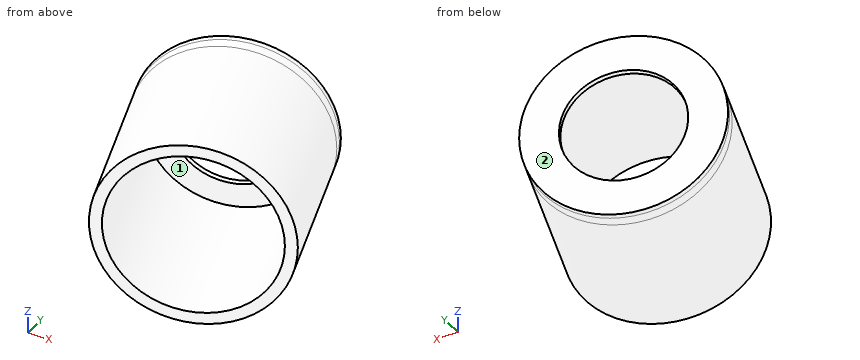
Autodesk Inventor part; units mm, degrees
ref_plane "YZ Plane" through (0, 0, 0) normal (1, 0, 0) x (0, 1, 0)
ref_plane "XZ Plane" through (0, 0, 0) normal (0, 1, 0) x (-1, 0, 0)
ref_plane "XY Plane" through (0, 0, 0) normal (0, 0, 1) x (1, 0, 0)
ref_plane "Work Plane2" through (-89.4914, 16.4002, -46.0725) normal (0, 0, 1) x (0.3299211, -0.9440085, 0)
sketch "Sketch3" plane through (-89.4914, 16.4002, -46.0725) normal (0, 0, 1) x (0.3299211, -0.9440085, 0)
  line L0 (142.5, 12.3) -> (142.5, -12.3)
  line L1 (142.35, 11.9681) -> (142.35, -12.4873)
  point P0 (45.0071, 79.0699)
  dimension "d3" = 0.15
sketch "Sketch2" plane through (-89.4914, 16.4002, -46.0725) normal (0, 0, 1) x (0.3299211, -0.9440085, 0)
  line L0 (144.2, -14) -> (171.4, -14)
  line L1 (142.5, -12.3) -> (142.5, 11.0344)
  line L2 (130, 22) -> (130, -22)
  line L3 (144.2, 16.15) -> (171.4, 16.15)
  line L4 (171.4, 16.15) -> (171.4, 14.15)
  line L5 (144.2, 14.15) -> (171.4, 14.15)
  line L6 (156.1685, 0) -> (84.745, 0) construction
  line L7 (144.2, 14.15) -> (142.35, 14.15)
  line L8 (142.35, 16.15) -> (144.2, 16.15)
  line L9 (142.35, 11.9681) -> (142.35, -12.4873)
  line L10 (142.5, 14.15) -> (142.35, 14.15)
  line L11 (142.35, 14.15) -> (142.35, 16.15)
  line L12 (142.35, 16.15) -> (142.5, 16.15)
  point P0 (45.0071, 79.0699)
  dimension "d7" = 2
revolve "Revolution1" add sketch "Sketch2" angle 360 about axis through (-37.9682, -131.0241, -46.0725) along (-0.3299211, 0.9440085, 0)
sketch "Sketch4" plane through (-42.5272, -117.9794, -46.0725) normal (-0.3299211, 0.9440085, 0) x (0.9440085, 0.3299211, 0)
  circle A0 centre (0, 0) radius 10
  circle A1 centre (0, 0) radius 16.15
  point P0 (79.0699, -46.0725)
  dimension "d4" = 20
extrude "Extrusion2" add sketch "Sketch4" along normal blind 1
properties part number "motor_handler"
CAD build for the part. Positions are in the model's coordinates, mm. Face numbers are marked on the shaded views. Round coordinates to 2 decimals unless told otherwise and drop trailing zeros. Loops run counter-clockwise (first coordinate to the right, second up) from the corner with the lowest first, then second, coordinate; pieces in that order, holes last. Notation, with made-up numbers: (85.25, -10.75) - (124.25, -10.75) arc R13 cw to (124.25, 5.25) - close; hole circle Ø4 at (8, -4.5). An arc over 180 degrees is marked (long way). Put each result on its own line as item: value.
1. Two-plate mould, pull along X, no slides. Class the marked faces 1 and 2: released by +X, released by -X, zero draft, split by the parting line, or undercut.
Geometry check:
face 1: undercut
face 2: released by -X
2. Wall check: line 1 (Z direction, x = -36.5, y = -125); line 2 (Z direction, x = -36.5, y = -142.5); line 3 (X direction, y = -139.5, z = -39.5). Give the ranges that are in metal, low to high.
Geometry check:
line 1: -61.87 to -59.81, -32.33 to -30.28
line 2: -62.04 to -60.02, -32.13 to -30.1
line 3: -50.63 to -48.28, -21.73 to -19.38
3. Pin check, flat tips, straight feed: P1, Ø1.5, axis at y = -129, z = -37, coming from the +X side; P2, Ø12, axis at x = -36, z = -39, coming from the +Y side; P3, Ø5, axis at x = -45.5, y = -126, coming from the +Z side. Stop position of each tip, or through.
Geometry check:
P1: x = -23.95
P2: y = -112.54
P3: z = -30.19
4. Slice it at A-A on z = -43. List the corners of the cut face in (x, y), and give its area (3 significant figures).
Geometry check:
outline: (-57.82, -122.27) - (-47.91, -150.63) - (-45.98, -149.96) - (-55.57, -122.54) - (-51.51, -121.12) - (-51.84, -120.18) - close; (-33.87, -113.9) - (-33.54, -114.84) - (-29.49, -113.42) - (-19.9, -140.85) - (-17.98, -140.17) - (-27.89, -111.8) - close
area: 131 mm²
5. Slice it at D-D on z = -33. List the corners of the cut face in (x, y), and give its area (3 significant figures).
Geometry check:
outline: (-51.81, -120.16) - (-50.87, -122.85) - (-41.9, -148.53) - (-38.06, -147.19) - (-47.64, -119.77) - (-37.41, -116.19) - (-27.83, -143.62) - (-23.99, -142.27) - (-33.9, -113.91) - close
area: 255 mm²
6. Slice it at B-B on z = -59. List the corners of the cut face in (x, y).
Geometry check:
outline: (-52, -120.23) - (-51.05, -122.92) - (-42.08, -148.6) - (-38.37, -147.3) - (-47.96, -119.88) - (-37.1, -116.08) - (-27.51, -143.5) - (-23.8, -142.21) - (-33.72, -113.84) - close
7. Slice it at C-C on z = -49. List the corners of the cut face in (x, y).
Geometry check:
outline: (-57.85, -122.28) - (-47.94, -150.64) - (-46.01, -149.97) - (-55.6, -122.55) - (-51.55, -121.13) - (-51.88, -120.19) - close; (-33.83, -113.88) - (-33.5, -114.82) - (-29.46, -113.41) - (-19.87, -140.84) - (-17.95, -140.16) - (-27.86, -111.8) - close
